Part model, mm, in its own coordinate system. Face numbers are marked on the shaded views. A direction names the side the tool comes from. Round coordinates to 2 decimals unless told otherwise and drop trailing zeros. Write each loop counter-clockwise with the first axis right and the second up, starting at its lowest first coordinate (ties: lowest second). Pieces come first, ordered by that corner, then holes.
1) Saw through at A-A on z = 26. Write the cut outline in (x, y), and give its area (3 significant figures).
2) Flat gauge pins, fed straight in: pin 1 (17 mm diameter, centred on y = -190, z = 52, fed in from +X); pin 2 (3 mm diameter, centred on y = -110, z = 46.5, fed in from -X); pin 3 (17 mm diameter, centred on x = -20.5, y = -184.5, fed in from -Z). Where does each tip first touch, or does it go through?
3) Pull direction X, two halves, no side cores. Call the marked faces 4, 5 and 6: +X half, -X half, draft (parallel to the pull), parting line (faces both ways), or undercut.
4) Drill centre lines: L1, parallel to Y at x = 13, z = 90; L2, parallel to Z at x = 22.5, y = -173.5; L3, parallel to Z at x = 46.5, y = 201.5. Where is each one in solid material? Low to high.
5) Saw through at B-B on x = -18.5. Write the cut outline in (y, z).
6) Which spindle directions (+Z, -Z, +X, -X, +Y, -Y) get a long thin tool onto all of the face, cutting with end or side? Do the marked faces 1, 2 and 3. Say none if no direction does.
7) Saw through at D-D on z = -7.5. Write the cut outline in (x, y).
8) Saw through at C-C on y = 68.5. Write the cut outline in (x, z).
```python
from build123d import *

# Parameters (mm, degrees)
BOSS_EXTRUDE1_DEPTH = 100
SKETCH3_W           = 200
SKETCH3_H           = 150
BOSS_EXTRUDE2_DEPTH = 75
CUT_EXTRUDE2_DEPTH  = 126
SKETCH6_W           = 140
SKETCH6_H           = 60
BOSS_EXTRUDE3_DEPTH = 100
SKETCH7_W           = 132
SKETCH7_H           = 92
CUT_EXTRUDE3_DEPTH  = 56


with BuildPart() as part:
    # Sketch2 → Boss-Extrude1 (new body)
    with BuildSketch(Plane.XY):
        Polygon((-50, 225), (50, 225), (100, -225), (-100, -225), align=None)
    extrude(amount=BOSS_EXTRUDE1_DEPTH)

    # Sketch3 → Boss-Extrude2 (add)
    with BuildSketch(Plane.XZ.offset(225)):
        with Locations((0, 50)):
            Rectangle(SKETCH3_W, SKETCH3_H)
    extrude(amount=BOSS_EXTRUDE2_DEPTH)

    # Sketch5 → Cut-Extrude2 (cut, through all)
    with BuildSketch(Plane(origin=(0, 0, 0), x_dir=(-1, 0, 0), z_dir=(0, 0, -1))):
        Polygon((-40.988033026, 125), (40.988033026, 125), (79.876921915, -225), (-79.876921915, -225), align=None)
    extrude(amount=-CUT_EXTRUDE2_DEPTH, mode=Mode.SUBTRACT)

    # Sketch6 → Boss-Extrude3 (add)
    with BuildSketch(Plane(origin=(0, 0, 0), x_dir=(-1, 0, 0), z_dir=(0, 0, -1))):
        with Locations((0, -195)):
            Rectangle(SKETCH6_W, SKETCH6_H)
    extrude(amount=-BOSS_EXTRUDE3_DEPTH)

    # Sketch7 → Cut-Extrude3 (cut)
    with BuildSketch(Plane(origin=(0, -165, 0), x_dir=(1, 0, 0), z_dir=(0, 1, 0))):
        with Locations((0, -50)):
            Rectangle(SKETCH7_W, SKETCH7_H)
    extrude(amount=-CUT_EXTRUDE3_DEPTH, mode=Mode.SUBTRACT)


solid = part.part
```
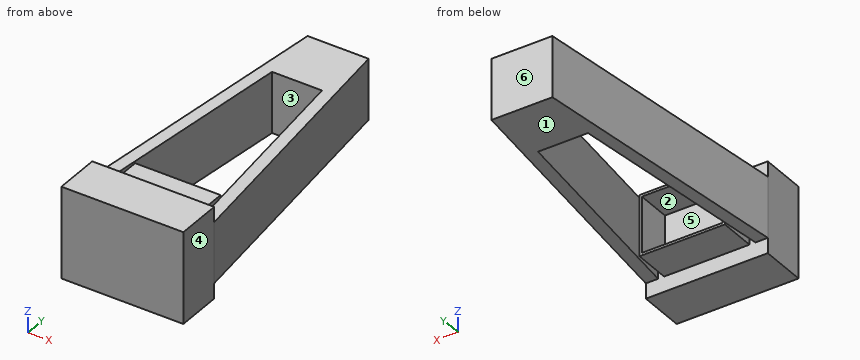
Completed:
1. outline: (-100, -300) - (100, -300) - (100, -225) - (50, 225) - (-50, 225) - (-100, -225) - close; hole (-79.88, -225) - (-70, -225) - (-70, -165) - (-66, -165) - (-66, -221) - (66, -221) - (66, -165) - (70, -165) - (70, -225) - (79.88, -225) - (40.99, 125) - (-40.99, 125) - close
1. area: 41,200 mm2
2. pin 1: stops at x = 97.06
2. pin 2: stops at x = -87.39
2. pin 3: stops at z = 0
3. face 4: +X half
3. face 5: undercut
3. face 6: draft
4. L1: y = -300 to -221, 125 to 225
4. L2: z = 0 to 4, 96 to 100
4. L3: z = 0 to 100
5. outline: (-300, -25) - (-225, -25) - (-225, 0) - (-165, 0) - (-165, 4) - (-221, 4) - (-221, 96) - (-165, 96) - (-165, 100) - (-225, 100) - (-225, 125) - (-300, 125) - close; (125, 0) - (225, 0) - (225, 100) - (125, 100) - close
6. face 1: -Z, +X, -X, +Y
6. face 2: none
6. face 3: +Z, -Z
7. outline: (-100, -300) - (100, -300) - (100, -225) - (-100, -225) - close
8. outline: (-67.39, 0) - (-47.27, 0) - (-47.27, 100) - (-67.39, 100) - close; (47.27, 0) - (67.39, 0) - (67.39, 100) - (47.27, 100) - close
